The drawing under review shows one solid part. Ordinate dimensions are in mm from its lowest x, y, z. A direction names the side the tool comes from. Coordinates: 2 decimals unless noted, no trailing zeros. Write each loop counter-clockwise with the first axis right and the second up, starting at its lowest first coordinate (ties: lowest second). Pieces come first, ordered by that corner, then holes. Notation, with made-up numbers: (5, 66.5) -> (18, 66.5) arc R20 ccw to (18, 100.5) -> close; hole circle Ø4 at (21, 27.5). An arc over 180 degrees is marked (long way). One line per item, written item: value. Start each with the question number.
1) Machinability: for the marked faces 1 and 2, which of the approach directions +Z, -Z, +X, -X, +Y, -Y give a long, thin tool a straight path to every point of the face, cutting with its end or side? Answer none if there is none.
2) Add section A-A (x = 89). State the section outline as (y, z) points, and give its area (3 significant figures).
3) For probe 1 along Z at (x, y) = (7.5, 25.5); probe 2 along Z at (x, y) = (92.5, 9); probe 3 along X at (y, z) = (5, 37), list the stretches that pass through material, from the lowest coordinate up. Write a range as from..to.
4) Mouldability with a two-part tool opening along Z and no side actions: class the marked faces 3, 4 and 5 as released by +Z, released by -Z, zero draft, split by the parting line, or undercut.
5) Add section B-B (z = 38.5). State the section outline as (x, y) points.
6) Add section C-C (y = 40). State the section outline as (x, z) points, and give its area (3 significant figures).
7) For pin 1 Ø4 at (x, z) = (7.5, 7.5) entering from -Y, flat-tipped, find the tip position at first contact; note if it passes through.
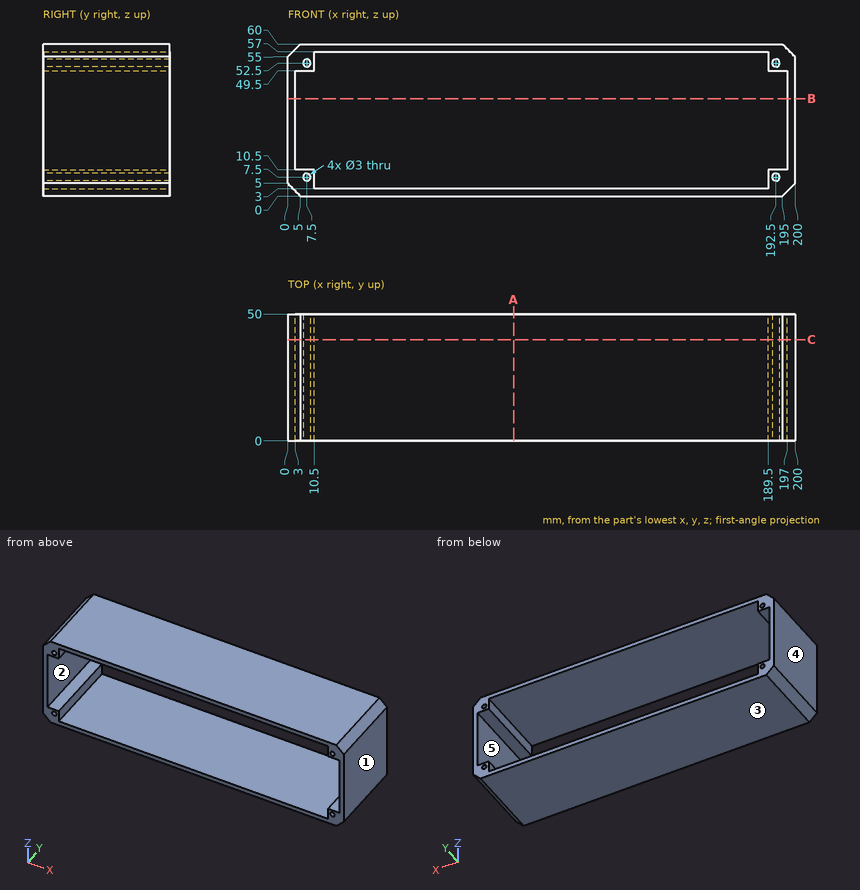
Numbers:
1. face 1: +Z, -Z, +X, +Y, -Y
1. face 2: +Y, -Y
2. outline: (0, 0) -> (50, 0) -> (50, 3) -> (0, 3) -> close; (0, 57) -> (50, 57) -> (50, 60) -> (0, 60) -> close
2. area: 300 mm²
3. probe 1: 0..6, 9..10.5, 49.5..51, 54..60
3. probe 2: 0..3, 57..60
3. probe 3: 0..3, 197..200
4. face 3: released by -Z
4. face 4: zero draft
4. face 5: undercut
5. outline: (0, 0) -> (3, 0) -> (3, 50) -> (0, 50) -> close; (197, 0) -> (200, 0) -> (200, 50) -> (197, 50) -> close
6. outline: (0, 5) -> (5, 0) -> (195, 0) -> (200, 5) -> (200, 55) -> (195, 60) -> (5, 60) -> (0, 55) -> close; hole (3, 10.5) -> (10.5, 10.5) -> (10.5, 3) -> (189.5, 3) -> (189.5, 10.5) -> (197, 10.5) -> (197, 49.5) -> (189.5, 49.5) -> (189.5, 57) -> (10.5, 57) -> (10.5, 49.5) -> (3, 49.5) -> close; hole circle Ø3 at (7.5, 7.5); hole circle Ø3 at (7.5, 52.5); hole circle Ø3 at (192.5, 7.5); hole circle Ø3 at (192.5, 52.5)
6. area: 1,670 mm²
7. pin 1: y = 0
